```python
from build123d import *

# Parameters (mm, degrees)
BOSS_EXTRUDE1_DEPTH                             = 17.45
CSK_FOR_M4_FLAT_HEAD_MACHINE_SCREW1_D           = 4.3
CSK_FOR_M4_FLAT_HEAD_MACHINE_SCREW1_CSINK_D     = 9.4
CSK_FOR_M4_FLAT_HEAD_MACHINE_SCREW1_CSINK_ANGLE = 90
SKETCH24_W                                      = 4.699
SKETCH24_H                                      = 41.40401941


with BuildPart() as part:
    # Sketch1 → Boss-Extrude1 (new body, symmetric)
    with BuildSketch(Plane.XY):
        with BuildLine():
            Line((-21.45, -10.95), (21.45, -10.95))
            ThreePointArc((21.45, -10.95), (23.217766953, -10.217766953), (23.95, -8.45))
            Line((23.95, -8.45), (23.95, 8.45))
            ThreePointArc((23.95, 8.45), (23.217766953, 10.217766953), (21.45, 10.95))
            Line((21.45, 10.95), (-21.45, 10.95))
            ThreePointArc((-21.45, 10.95), (-23.217766953, 10.217766953), (-23.95, 8.45))
            Line((-23.95, 8.45), (-23.95, -8.45))
            ThreePointArc((-23.95, -8.45), (-23.217766953, -10.217766953), (-21.45, -10.95))
        make_face()
    extrude(amount=BOSS_EXTRUDE1_DEPTH, both=True)

    # CSK for M4 Flat Head Machine Screw1 (through all)
    with Locations(Plane.XY.offset(17.45)):
        with Locations((-16.388274302, -5.782084253), (16.388274302, 5.782084253)):
            CounterSinkHole(CSK_FOR_M4_FLAT_HEAD_MACHINE_SCREW1_D / 2, CSK_FOR_M4_FLAT_HEAD_MACHINE_SCREW1_CSINK_D / 2, counter_sink_angle=CSK_FOR_M4_FLAT_HEAD_MACHINE_SCREW1_CSINK_ANGLE)

    # Sketch24 → Hosel Diameter (revolve, cut)
    with BuildSketch(Plane(origin=(-1.212269458, -0.441229999, 0), x_dir=(0, 0, -1), z_dir=(0.939692621, 0.342020143, 0))):
        with Locations((2.2345, -1.146750947)):
            Rectangle(SKETCH24_W, SKETCH24_H)
    revolve(axis=Axis((-7.900561861, 17.934702354, 0.115), (0.342020143, -0.939692621, 0)), mode=Mode.SUBTRACT)


solid = part.part
```
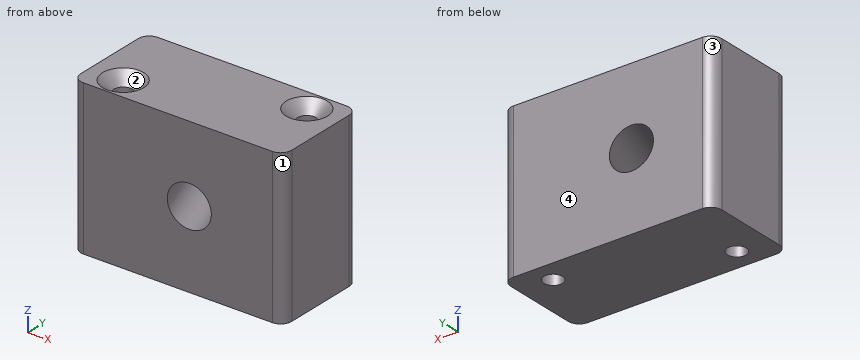
CAD build for the part. Positions are in the model's coordinates, mm. Face numbers are marked on the shaded views. Give positions to 0.01 mm unless a question says otherwise; leave off trailing zeros. Order: outer loops, then holes, each group sorted by start corner. A loop starts at its lowest first (then second) coordinate and runs counter-clockwise, first axis right, second up.
(1) Saw through at A-A, the plane z = -3.5. Give the cut face in (x, y), then the cut area to 3 significant figures.
(2) Mould opens along X. For the marked faces 1, 2, 3 and 4 say: released by +X, released by -X, zero draft, split by the parting line, or undercut.
(3) Drill centre lines: L1, parallel to X at y = -5.75, z = 10.5; L2, parallel to X at y = -7.75, z = -1; L3, parallel to X at y = -7.5, z = -14. Where is each one in solid material? Low to high.
(4) Saw through at B-B, the plane y = -4.25. State how many separate pieces and enclosed holes the cut face has, then the cut area to 3 significant figures.
(5) Flat gauge pins, fed straight in: pin 1 (5 mm diameter, centred on x = 17.5, y = 4, fed in from +Z); pin 2 (7 mm diameter, centred on x = -16.39, y = -5.78, fed in from +Z). Where does each tip first touch, or does it go through?
Results found:
1. outline: (-23.95, -8.45) arc R2.5 ccw to (-21.45, -10.95) - (-0.58, -10.95) - (-8.55, 10.95) - (-21.45, 10.95) arc R2.5 ccw to (-23.95, 8.45) - close; (-2.16, 10.95) - (5.81, -10.95) - (21.45, -10.95) arc R2.5 ccw to (23.95, -8.45) - (23.95, 8.45) arc R2.5 ccw to (21.45, 10.95) - close; hole circle Ø4.3 at (-16.39, -5.78); hole circle Ø4.3 at (16.39, 5.78)
1. area: 875 mm2
2. face 1: released by +X
2. face 2: undercut
2. face 3: released by -X
2. face 4: zero draft
3. L1: x = -23.95 to -18.54, -14.24 to 23.95
3. L2: x = -23.95 to -17.25, -15.52 to -3.41, 6.31 to 23.95
3. L3: x = -23.95 to -17.68, -15.1 to 23.95
4. separate pieces: 2
4. enclosed holes: 1
4. area: 1,480 mm2
5. pin 1: stops at z = 17.35
5. pin 2: stops at z = 16.25
